```python
from build123d import *

# Parameters (mm, degrees)
SKETCH1_W           = 100
SKETCH1_H           = 50
BOSS_EXTRUDE1_DEPTH = 10
FILLET1_R           = 10
SKETCH2_R           = 2.1
CUT_EXTRUDE1_DEPTH  = 10


with BuildPart() as part:
    # Sketch1 → Boss-Extrude1 (new body)
    with BuildSketch(Plane(origin=(0, 0, 0), x_dir=(1, 0, 0), z_dir=(0, 1, 0))):
        Rectangle(SKETCH1_W, SKETCH1_H)
    extrude(amount=BOSS_EXTRUDE1_DEPTH)

    # Fillet1
    fillet1_edges = [part.edges().sort_by_distance(p)[0] for p in [
        (-50, 5, -25),
        (50, 5, -25),
        (50, 5, 25),
        (-50, 5, 25),
    ]]
    fillet(fillet1_edges, radius=FILLET1_R)

    # Sketch2 → Cut-Extrude1 (cut)
    with BuildSketch(Plane(origin=(0, 10, 0), x_dir=(1, 0, 0), z_dir=(0, 1, 0))):
        with Locations(Location((-42.132384366, 18.438889303, 0), (0, 0, 270))):
            Circle(SKETCH2_R)
        with Locations(Location((42.132384366, 18.438889303, 0), (0, 0, 270))):
            Circle(SKETCH2_R)
        with Locations(Location((42.132384366, -18.438889303, 0), (0, 0, 270))):
            Circle(SKETCH2_R)
        with Locations(Location((-42.132384366, -18.438889303, 0), (0, 0, 270))):
            Circle(SKETCH2_R)
    extrude(amount=-CUT_EXTRUDE1_DEPTH, mode=Mode.SUBTRACT)


solid = part.part
```
Model file for the job. Use its own axes, mm. Give positions to 0.01 mm unless a question says otherwise; leave off trailing zeros. Loops run counter-clockwise (first coordinate to the right, second up) from the corner with the lowest first, then second, coordinate; pieces in that order, holes last. Notation, with made-up numbers: (78.5, 8.5) - (100.5, 8.5) arc R24 ccw to (100.5, 29.5) - close; hole circle Ø5 at (-1, -38.5). An arc over 180 degrees is marked (long way). One line per item, written item: value. Start each with the question number.
1. Probe L1, parallel to X at y = 9.5, z = -16; L2, parallel to X at y = 5.75, z = -22. List the from-to ranges inside material, lowest first. Write a range as from..to.
2. Pin check, flat tips, straight feed: pin 1 (2.5 mm diameter, centred on x = -42.13, z = 18.44, fed in from -Y); pin 2 (1.5 mm diameter, centred on y = 8, z = -19, fed in from -X). Stop position of each tip, or through.
3. Pull direction Z, two halves, no side cores. Call faces 1 (the cylindrical face through (-43.995, 5.07, -17.47)), 2 (the flat face through (-1, 5, -25)), 3 (the flat face through (-1, 0, 0)): pulls with the +Z half, pulls with the -Z half, needs draft (parallel to the pull), parting line crosses it, or undercut.
4. Slice it at A-A (y = 1.75). List the corners of the cut face in (x, z), plus the area to 3 significant figures.
Solution:
1. L1: x = -49.95..49.95
1. L2: x = -47.14..47.14
2. pin 1: passes through
2. pin 2: stops at x = -49.46
3. face 1: undercut
3. face 2: pulls with the -Z half
3. face 3: needs draft
4. outline: (-50, -15) arc R10 ccw to (-40, -25) - (40, -25) arc R10 ccw to (50, -15) - (50, 15) arc R10 ccw to (40, 25) - (-40, 25) arc R10 ccw to (-50, 15) - close; hole circle Ø4.2 at (-42.13, -18.44); hole circle Ø4.2 at (-42.13, 18.44); hole circle Ø4.2 at (42.13, -18.44); hole circle Ø4.2 at (42.13, 18.44)
4. area: 4,860 mm^2
